The model under review builds one solid part; all positions refer to its coordinate system, in mm. Face numbers are marked on the shaded views. A direction names the side the tool comes from. Give positions to 0.01 mm unless a question says otherwise; leave off trailing zeros. Loops run counter-clockwise (first coordinate to the right, second up) from the corner with the lowest first, then second, coordinate; pieces in that order, holes last. Notation, with made-up numbers: (9.25, 43.25) - (36.25, 43.25) arc R31 cw to (36.25, 77.25) - close; hole circle Ø7 at (-12.75, 56). An arc over 180 degrees is marked (long way). Return JSON: item names as keys, results as strings. Group by question number.
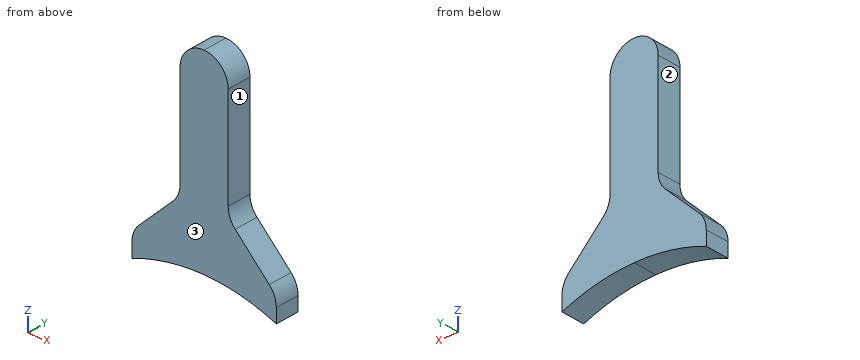
from build123d import *

# Parameters (mm, degrees)
BOSS_EXTRUDE1_DEPTH = 12.7
FILLET1_R           = 12.7


with BuildPart() as part:
    # Sketch1 → Boss-Extrude1 (new body)
    with BuildSketch(Plane(origin=(0, 0, 0), x_dir=(1, 0, 0), z_dir=(0, 1, 0))):
        with BuildLine():
            Line((0, -101.6), (0, -203.2))
            Line((0, -203.2), (12.7, -203.2))
            Line((12.7, -203.2), (12.7, -132.285720786))
            Line((12.7, -132.285720786), (38.1, -106.885720786))
            Line((38.1, -106.885720786), (38.1, -94.185720786))
            ThreePointArc((38.1, -94.185720786), (19.407353866, -99.729206434), (0, -101.6))
        make_face()
    extrude(amount=BOSS_EXTRUDE1_DEPTH)

    # Fillet1
    fillet1_edges = [part.edges().sort_by_distance(p)[0] for p in [
        (38.1, 6.35, 106.885720786),
        (12.7, 6.35, 132.285720786),
        (12.7, 6.35, 203.2),
    ]]
    fillet(fillet1_edges, radius=FILLET1_R - 0.0001)  # a hair under: the kernel refuses the full size

    # Mirror1: part across plane


with BuildPart() as part_1:
    add(part.part)
    add(part.part.mirror(Plane(origin=(0, 12.7, 101.6), x_dir=(0, 0, 1), z_dir=(1, 0, 0))))


solid = part_1.part
Item 1: Take a section at C-C (x = 30.5). State the section outline as (y, z) points.
Item 2: For L1, parallel to X at y = 10.5, z = 145; L2, parallel to X at y = 0.5, z = 134; L3, parallel to Z at x = 15.5, y = 11, list the stretches that pass through material, from the lowest coordinate up. Write a range as from..to.
Item 3: Take a section at B-B (z = 143). State the section outline as (x, y) points, then the cut area to 3 significant figures.
Item 4: Tool access review of the marked faces 1, 2 and 3: name each direction out of +Z, -Z, +X, -X, +Y, -Y from which nothing blocks a thin tool from reaching the whole face with its end or side.
Item 5: For P1, Ø4, axis at y = 4.5, z = 172.5, coming from the +X side; P2, Ø1, axis at y = 10.5, z = 179, coming from the -X side; P3, Ø1, axis at x = -30, y = 6, coming from the -Z side, all flat-tipped, find the tip position at first contact; note any pin that passes through.
Check sheet entries:
{
 "1": {"outline": "(0, 96.91) - (12.7, 96.91) - (12.7, 114.49) - (0, 114.49) - close"},
 "2": {"L1": "x = -12.7..12.7", "L2": "x = -13.21..13.21", "L3": "z = 100.41..129.59"},
 "3": {"outline": "(-12.7, 0) - (12.7, 0) - (12.7, 12.7) - (-12.7, 12.7) - close", "area": "323 mm^2"},
 "4": {"face 1": "+Z, +X, +Y, -Y", "face 2": "+Z, -X, +Y, -Y", "face 3": "+Z, -Z, +X, -X, -Y"},
 "5": {"P1": "stops at x = 12.7", "P2": "stops at x = -12.7", "P3": "stops at z = 96.91"}
}
